Build history of the part. All positions in model axes, mm. Give positions to 0.01 mm unless a question says otherwise; leave off trailing zeros. Loops run counter-clockwise (first coordinate to the right, second up) from the corner with the lowest first, then second, coordinate; pieces in that order, holes last. Notation, with made-up numbers: (-36, 41) -> (2, 41) arc R34 cw to (2, 71) -> close; hole circle Ø8 at (22, 32). An arc over 180 degrees is marked (long way). Answer as a JSON object with one key per item and string values. Group by question number.
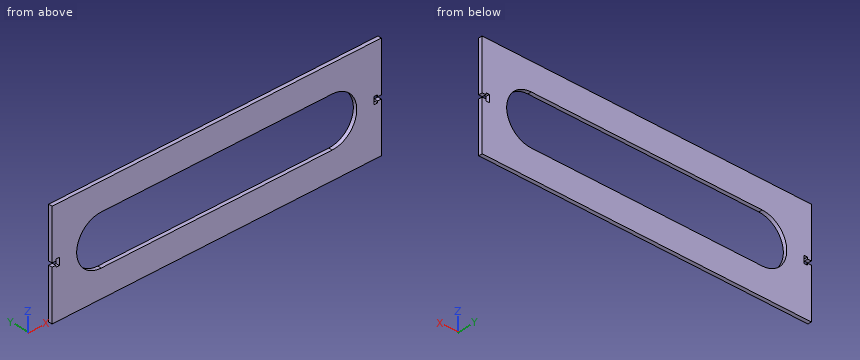
from build123d import *

# Parameters (mm, degrees)
SALIENTE_EXTRUIR2_DEPTH = 3


with BuildPart() as part:
    # Croquis1 → Saliente-Extruir2 (new body)
    with BuildSketch(Plane(origin=(0, 0, 0), x_dir=(1, 0, 0), z_dir=(0, 1, 0))):
        Polygon((134, -42), (-134, -42), (-134, -1.5), (-131, -1.5), (-131, -3), (-128, -3), (-128, 3), (-131, 3), (-131, 1.5), (-134, 1.5), (-134, 42), (134, 42), (134, 1.5), (131, 1.5), (131, 3), (128, 3), (128, -3), (131, -3), (131, -1.5), (134, -1.5), align=None)
        with BuildLine():
            Line((94, -20), (-94, -20))
            ThreePointArc((-94, -20), (-114, 0), (-94, 20))
            Line((-94, 20), (94, 20))
            ThreePointArc((94, 20), (114, 0), (94, -20))
        make_face(mode=Mode.SUBTRACT)
    extrude(amount=SALIENTE_EXTRUIR2_DEPTH)


solid = part.part
(1) Saw through at A-A on x = -13.5. List the corners of the cut face in (y, z).
(2) Saw through at C-C on z = -16.5. List the corners of the cut face in (x, y).
(3) Probe line 1 along Z through (x, y) = (42, 2); line 2 along Z through (x, y) = (99.5, 0.5); line 3 along X through (y, z) = (0.95, -14). List the from-to ranges inside material, lowest first. Write a range as [from, to].
(4) Saw through at B-B on y = 1.75. List the corners of the cut face in (x, z), plus the area to 3 significant figures.
Calculated:
{
 "1": {"outline": "(0, -42) -> (3, -42) -> (3, -20) -> (0, -20) -> close; (0, 20) -> (3, 20) -> (3, 42) -> (0, 42) -> close"},
 "2": {"outline": "(-134, 0) -> (-105.3, 0) -> (-105.3, 3) -> (-134, 3) -> close; (105.3, 0) -> (134, 0) -> (134, 3) -> (105.3, 3) -> close"},
 "3": {"line 1": "z = [-42, -20], [20, 42]", "line 2": "z = [-42, -19.23], [19.23, 42]", "line 3": "x = [-134, -108.28], [108.28, 134]"},
 "4": {"outline": "(-134, -42) -> (134, -42) -> (134, -1.5) -> (131, -1.5) -> (131, -3) -> (128, -3) -> (128, 3) -> (131, 3) -> (131, 1.5) -> (134, 1.5) -> (134, 42) -> (-134, 42) -> (-134, 1.5) -> (-131, 1.5) -> (-131, 3) -> (-128, 3) -> (-128, -3) -> (-131, -3) -> (-131, -1.5) -> (-134, -1.5) -> close; hole (-94, -20) -> (94, -20) arc R20 ccw to (94, 20) -> (-94, 20) arc R20 ccw to start", "area": "13,700 mm^2"}
}
